Can you work these out from the model? Positions are in its coordinate system, mm. A direction names the side the tool comes from. Give positions to 0.01 mm unless a question says otherwise; leave off trailing zeros. Loops run counter-clockwise (first coordinate to the right, second up) from the corner with the lowest first, then second, coordinate; pieces in that order, holes last.
from build123d import *

# Parameters (mm, degrees)
F0_R     = 41.5
F1_DEPTH = 75
F2_R     = 32.5
F3_DEPTH = 70
F4_R     = 41.5
F4_R_2   = 37.5
F5_DEPTH = 70


with BuildPart() as f1:
    # F0 (on Top) → F1 (new body)
    with BuildSketch(Plane.XY):
        Circle(F0_R)
    extrude(amount=F1_DEPTH)

    # F2 (on face) → F3 (cut)
    with BuildSketch(Plane.XY.offset(75)):
        Circle(F2_R)
    extrude(amount=-F3_DEPTH, mode=Mode.SUBTRACT)

    # F4 (on face) → F5 (cut)
    with BuildSketch(Plane(origin=(0, 0, 0), x_dir=(1, 0, 0), z_dir=(0, 0, -1))):
        Circle(F4_R)
        Circle(F4_R_2, mode=Mode.SUBTRACT)
    extrude(amount=-F5_DEPTH, mode=Mode.SUBTRACT)


solid = f1.part
(1) Thinking about a two-plate mould opening in X: for faces 1 (the cylindrical face through (31, 9.76, 40.49)), 2 (the cylindrical face through (39.584, 12.465, 72.465)), 3 (the flat face through (-1, 1, 0)), which applies, pulls with the +X half, pulls with the -X half, needs draft (parallel to the pull), parting line crosses it, or undercut?
Returned:
face 1: undercut
face 2: parting line crosses it
face 3: needs draft
(2) Please list where these lines run through material, in increasing order: probe 1 along Y at (x, z) = (0, 40); probe 2 along Z at (x, y) = (36, 11); probe 3 along X at (y, z) = (-27.5, 71.5).
Returned:
probe 1: y = -37.5 to -32.5, 32.5 to 37.5
probe 2: z = 70 to 75
probe 3: x = -31.08 to -17.32, 17.32 to 31.08
(3) Suppose I cut it at A-A on z = 56. List the corners of the cut face in (x, y) for me, plus the area to 3 significant figures.
Returned:
outline: circle Ø75 at (0, 0); hole circle Ø65 at (0, 0)
area: 1,100 mm2
(4) Which directions (+Z, -Z, +X, -X, +Y, -Y) give clear straight access to the entire face, cutting with the end or side of a thin tool? Please do faces 4 (the flat face through (0, 0, 5)), 5 (the flat face through (-9, 37, 70)), 6 (the flat face through (-24.8, -21.3, 75)).
Returned:
face 4: +Z
face 5: -Z
face 6: +Z, +X, -X, +Y, -Y
(5) Will these pins go through, and if not, where does the flat tip stop? P1, Ø1.5, axis at x = -13.5, z = 20.5, coming from the -Y side; P2, Ø5, axis at y = -20, z = 19.5, coming from the +X side; P3, Ø1, axis at x = -22.5, y = -2, coming from the -Z side; P4, Ø1.5, axis at x = -3, z = 17.5, coming from the -Y side.
Returned:
P1: stops at y = -35.27
P2: stops at x = 33.17
P3: stops at z = 0
P4: stops at y = -37.43
(6) Suppose I cut it at B-B on y = 0. List the corners of the cut face in (x, z) for me.
Returned:
outline: (-41.5, 70) - (-37.5, 70) - (-37.5, 0) - (37.5, 0) - (37.5, 70) - (41.5, 70) - (41.5, 75) - (32.5, 75) - (32.5, 5) - (-32.5, 5) - (-32.5, 75) - (-41.5, 75) - close
